Here's the drawing with two shaded views (mm, measured from the low corner). I have some questions. Give positions to 0.01 mm unless a question says otherwise; leave off trailing zeros. Write each loop counter-clockwise with the first axis right and the second up, starting at its lowest first coordinate (ties: lowest second). Pieces come first, ordered by that corner, then holes. Notation, with made-up numbers: (1, -1.5) -> (22, -1.5) arc R27 ccw to (22, 22.5) -> close; hole circle Ø2 at (63.25, 66). An arc over 180 degrees is marked (long way). Put each result on its own line as item: value. Start each with the question number.
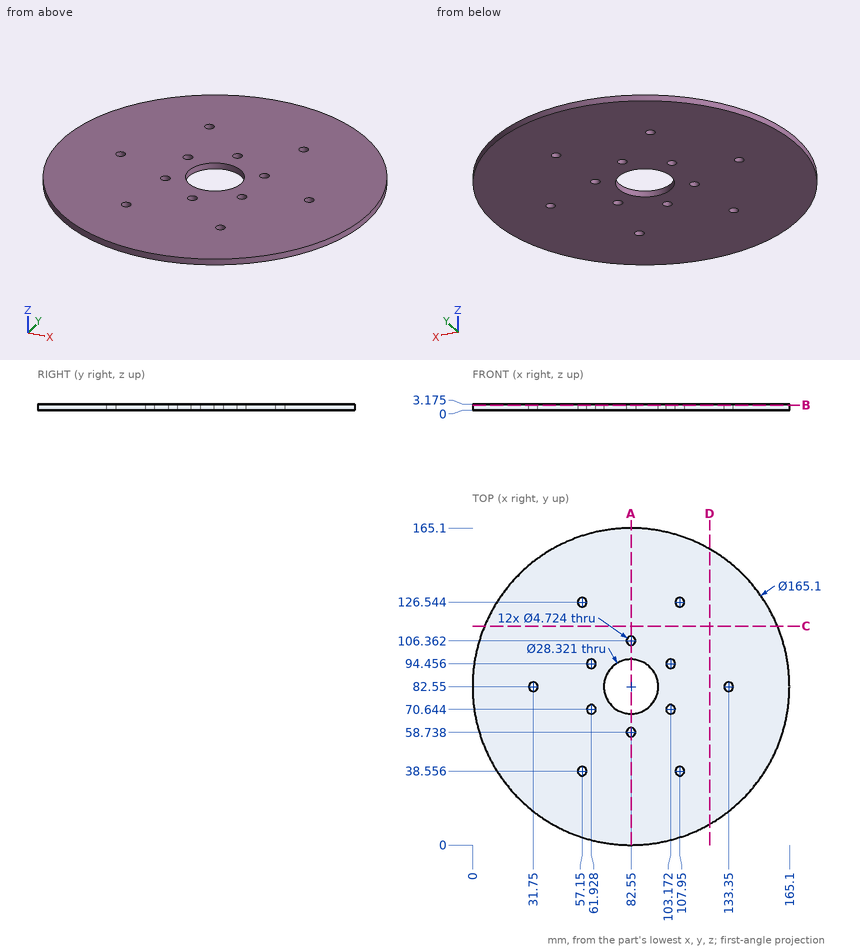
1) I'm going to push a flat-ended pin straight in: pin 1 Ø1 at (y, z) = (32.5, 1.5) entering from +X (1 decimal). Where does the tip first touch, or does it pass through?
2) I want a section at A-A, the plane x = 82.55. Write out the boundary of the cut face in (y, z) (1 decimal).
3) I want a section at D-D, the plane x = 123.5. Write out the boundary of the cut face in (y, z) (1 decimal), and give its area (3 significant figures).
4) I want a section at B-B, the plane z = 2.65. State how many separate pieces and enclosed holes the cut face has, and give its area (3 significant figures).
5) I need wall thicknesses on probe 1 along Y at (x, z) = (82.55, 2.2) (1 decimal); probe 2 along X at (y, z) = (128, 2.25); probe 3 along Y at (x, z) = (84, 0.4) (1 decimal). Which ranges of each line are inside material? Lowest first, please.
6) I want a section at C-C, the plane y = 114. Write out the boundary of the cut face in (x, z) (1 decimal).
Established:
1. pin 1: stops at x = 148.6
2. outline: (0, 0) -> (56.4, 0) -> (56.4, 3.2) -> (0, 3.2) -> close; (61.1, 0) -> (68.4, 0) -> (68.4, 3.2) -> (61.1, 3.2) -> close; (96.7, 0) -> (104, 0) -> (104, 3.2) -> (96.7, 3.2) -> close; (108.7, 0) -> (165.1, 0) -> (165.1, 3.2) -> (108.7, 3.2) -> close
3. outline: (10.9, 0) -> (154.2, 0) -> (154.2, 3.2) -> (10.9, 3.2) -> close
3. area: 455 mm2
4. separate pieces: 1
4. enclosed holes: 13
4. area: 20,600 mm2
5. probe 1: y = 0 to 56.4, 61.1 to 68.4, 96.7 to 104, 108.7 to 165.1
5. probe 2: x = 13.64 to 55.29, 59.01 to 106.09, 109.81 to 151.46
5. probe 3: y = 0 to 56.9, 60.6 to 68.5, 96.6 to 104.5, 108.2 to 165.1
6. outline: (6.2, 0) -> (158.9, 0) -> (158.9, 3.2) -> (6.2, 3.2) -> close
